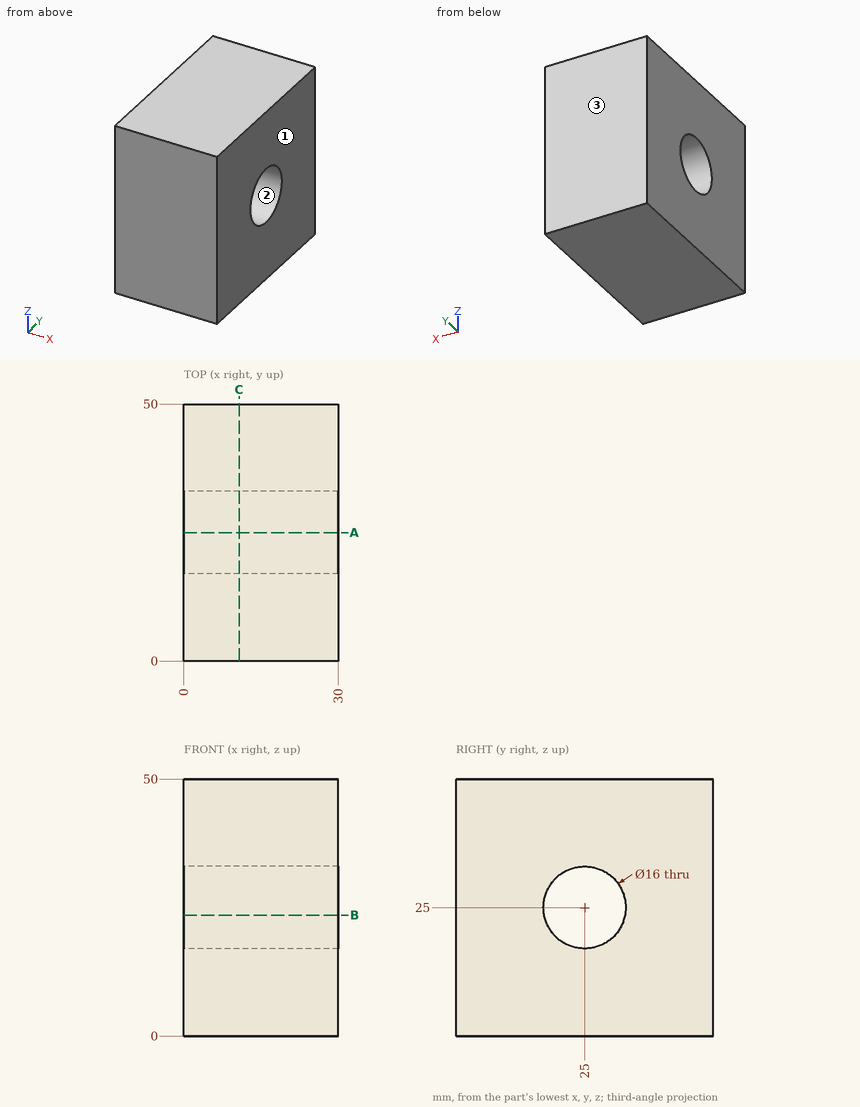
Design review of the part shown in the three views and the two pictorial views. Dimensions are in mm from the part's minimum x, y and z. Coordinates: 2 decimals unless noted, no trailing zeros. Loops run counter-clockwise (first coordinate to the right, second up) from the corner with the lowest first, then second, coordinate; pieces in that order, holes last.
Q1. The part is to be moulded in two halves that separate along Y. For the marked faces 1, 2 and 3, say which applies: +Y half, -Y half, draft (parallel to the pull), parting line (faces both ways), or undercut.
Reported:
face 1: draft
face 2: undercut
face 3: +Y half
Q2. We need section A-A on y = 25. State the section outline as (x, z) points, and give its area (3 significant figures).
Reported:
outline: (0, 0) - (30, 0) - (30, 17) - (0, 17) - close; (0, 33) - (30, 33) - (30, 50) - (0, 50) - close
area: 1,020 mm2
Q3. We need section C-C on x = 10.75. State the section outline as (y, z) points, and give its area (3 significant figures).
Reported:
outline: (0, 0) - (50, 0) - (50, 50) - (0, 50) - close; hole circle Ø16 at (25, 25)
area: 2,300 mm2
Q4. We need section B-B on z = 23.5. State the section outline as (x, y) points, and give its area (3 significant figures).
Reported:
outline: (0, 0) - (30, 0) - (30, 17.14) - (0, 17.14) - close; (0, 32.86) - (30, 32.86) - (30, 50) - (0, 50) - close
area: 1,030 mm2
Q5. To check wall thickness, follow line 1 (Y direction, x = 12.5, z = 25); line 2 (Z direction, x = 11.75, y = 31.5). State the ranges of each line that lie inside material, in increasing order.
Reported:
line 1: y = 0 to 17, 33 to 50
line 2: z = 0 to 20.34, 29.66 to 50
